```python
from build123d import *

# Parameters (mm, degrees)
SKETCH1_W           = 212.5
SKETCH1_H           = 339.725
SKETCH1_R           = 3.175
BOSS_EXTRUDE1_DEPTH = 3.175
CUT_EXTRUDE1_DEPTH  = 401.72360331
SKETCH3_R           = 4
CUT_EXTRUDE2_DEPTH  = 45.72
SKETCH4_R           = 4
CUT_EXTRUDE3_DEPTH  = 14.986


with BuildPart() as part:
    # Sketch1 → Boss-Extrude1 (new body)
    with BuildSketch(Plane(origin=(0, 0, 0), x_dir=(0, 0, -1), z_dir=(1, 0, 0))):
        with Locations((106.25, -169.8625)):
            Rectangle(SKETCH1_W, SKETCH1_H)
        with Locations((12.7, -12.7)):
            Circle(SKETCH1_R, mode=Mode.SUBTRACT)
        with Locations((199.8, -12.7)):
            Circle(SKETCH1_R, mode=Mode.SUBTRACT)
        with Locations((66.25, -35.2425)):
            Circle(SKETCH1_R, mode=Mode.SUBTRACT)
        with Locations((146.25, -35.2425)):
            Circle(SKETCH1_R, mode=Mode.SUBTRACT)
        with Locations((176.25, -57.8625)):
            Circle(SKETCH1_R, mode=Mode.SUBTRACT)
        with Locations((36.25, -57.8625)):
            Circle(SKETCH1_R, mode=Mode.SUBTRACT)
        with Locations((191.25, -104.5325)):
            Circle(SKETCH1_R, mode=Mode.SUBTRACT)
        with Locations((36.25, -169.8625)):
            Circle(SKETCH1_R, mode=Mode.SUBTRACT)
        with Locations((191.25, -169.8625)):
            Circle(SKETCH1_R, mode=Mode.SUBTRACT)
        with Locations((36.25, -281.8625)):
            Circle(SKETCH1_R, mode=Mode.SUBTRACT)
        with Locations((66.25, -304.4825)):
            Circle(SKETCH1_R, mode=Mode.SUBTRACT)
        with Locations((12.7, -327.025)):
            Circle(SKETCH1_R, mode=Mode.SUBTRACT)
        with Locations((199.8, -327.025)):
            Circle(SKETCH1_R, mode=Mode.SUBTRACT)
        with Locations((146.25, -304.4825)):
            Circle(SKETCH1_R, mode=Mode.SUBTRACT)
        with Locations(Location((191.25, -235.1925, 0), (0, 0, 180))):
            Circle(SKETCH1_R, mode=Mode.SUBTRACT)
    extrude(amount=BOSS_EXTRUDE1_DEPTH)

    # Sketch2 → Cut-Extrude1 (cut, through all)
    with BuildSketch(Plane(origin=(3.175, 0, 0), x_dir=(0, 0, -1), z_dir=(1, 0, 0))):
        with BuildLine():
            Line((165.85, -88.161695758), (165.85, -251.563304242))
            ThreePointArc((165.85, -251.563304242), (164.516472011, -257.22840036), (160.795934799, -261.703801323))
            Line((160.795934799, -261.703801323), (125.904065201, -288.012271))
            ThreePointArc((125.904065201, -288.012271), (122.183527989, -292.487671963), (120.85, -298.152768081))
            Line((120.85, -298.152768081), (120.85, -314.325))
            ThreePointArc((120.85, -314.325), (117.130256121, -323.305256121), (108.15, -327.025))
            Line((108.15, -327.025), (104.35, -327.025))
            ThreePointArc((104.35, -327.025), (95.369743879, -323.305256121), (91.65, -314.325))
            Line((91.65, -314.325), (91.65, -298.152768081))
            ThreePointArc((91.65, -298.152768081), (90.316472011, -292.487671963), (86.595934799, -288.012271))
            Line((86.595934799, -288.012271), (48.147303392, -259.022002919))
            ThreePointArc((48.147303392, -259.022002919), (44.532850149, -257.119362682), (40.501368593, -256.4625))
            Line((40.501368593, -256.4625), (25.4, -256.4625))
            ThreePointArc((25.4, -256.4625), (16.419743879, -252.742756121), (12.7, -243.7625))
            Line((12.7, -243.7625), (12.7, -207.9625))
            ThreePointArc((12.7, -207.9625), (16.419743879, -198.982243879), (25.4, -195.2625))
            Line((25.4, -195.2625), (48.95, -195.2625))
            ThreePointArc((48.95, -195.2625), (57.930256121, -191.542756121), (61.65, -182.5625))
            Line((61.65, -182.5625), (61.65, -157.1625))
            ThreePointArc((61.65, -157.1625), (57.930256121, -148.182243879), (48.95, -144.4625))
            Line((48.95, -144.4625), (25.4, -144.4625))
            ThreePointArc((25.4, -144.4625), (16.419743879, -140.742756121), (12.7, -131.7625))
            Line((12.7, -131.7625), (12.7, -95.9625))
            ThreePointArc((12.7, -95.9625), (16.419743879, -86.982243879), (25.4, -83.2625))
            Line((25.4, -83.2625), (40.501368593, -83.2625))
            ThreePointArc((40.501368593, -83.2625), (44.532850149, -82.605637318), (48.147303392, -80.702997081))
            Line((48.147303392, -80.702997081), (86.595934799, -51.712729))
            ThreePointArc((86.595934799, -51.712729), (90.316472011, -47.237328037), (91.65, -41.572231919))
            Line((91.65, -41.572231919), (91.65, -25.4))
            ThreePointArc((91.65, -25.4), (95.369743879, -16.419743879), (104.35, -12.7))
            Line((104.35, -12.7), (108.15, -12.7))
            ThreePointArc((108.15, -12.7), (117.130256121, -16.419743879), (120.85, -25.4))
            Line((120.85, -25.4), (120.85, -41.572231919))
            ThreePointArc((120.85, -41.572231919), (122.183527989, -47.237328037), (125.904065201, -51.712729))
            Line((125.904065201, -51.712729), (160.795934799, -78.021198677))
            ThreePointArc((160.795934799, -78.021198677), (164.516472011, -82.49659964), (165.85, -88.161695758))
        make_face()
    extrude(amount=-CUT_EXTRUDE1_DEPTH, mode=Mode.SUBTRACT)

    # Sketch3 → Cut-Extrude2 (cut)
    with BuildSketch(Plane.ZY):
        with Locations((-353.343139499, -302.41374809)):
            Circle(SKETCH3_R)
    extrude(amount=-CUT_EXTRUDE2_DEPTH, mode=Mode.SUBTRACT)

    # Sketch4 → Cut-Extrude3 (cut)
    with BuildSketch(Plane.ZY):
        with Locations((-76.9625, -23.613540107)):
            Circle(SKETCH4_R)
    extrude(amount=-CUT_EXTRUDE3_DEPTH, mode=Mode.SUBTRACT)


solid = part.part
```
Source: CAD feature listing. Evaluate the final solid. Frame: model axes, mm. A direction names the side the tool comes from. Coordinates: 2 decimals unless noted, no trailing zeros. Loops run counter-clockwise (first coordinate to the right, second up) from the corner with the lowest first, then second, coordinate; pieces in that order, holes last. Notation, with made-up numbers: (-35, 51.25) -> (-2, 51.25) arc R12 ccw to (-2, 55.25) -> close; hole circle Ø10 at (83.25, 5). An arc over 180 degrees is marked (long way). One line per item, written item: value. Start each with the question number.
Q1. Set-up query: faces 1 (the face through (1.61, -16.32, -117.03)), 2 (the face through (0, -167, -58)). Return all of +Z, -Z, +X, -X, +Y, -Y with unobstructed straight access to the full face (end or side cutting, diameter ignored); none if empty.
Q2. Section query B-B, the plane x = 1.3. Give the number of separate pieces and of enclosed holes in the cut face, and give its area (3 significant figures).
Q3. Mould query, pull axis Z, two halves, no side actions, for faces 3 (the face through (1.57, -104.39, -188.08)), 4 (the face through (3.175, -167, -58)). Classes: pulls with the +Z half, pulls with the -Z half, needs draft (parallel to the pull), parting line crosses it, or undercut.
Q4. Contact query for a flat-ended pin moving along its axis: P1, Ø4, axis at y = -281.86, z = -36.25, coming from the -X side. Output: stop coordinate, or through.
Q5. Section query A-A, the plane z = -130.5. Return the cut outline in (x, y) (3 decimals), and give its area (3 significant figures).
Q6. Line query: line 1 along Y through (x, z) = (1.6, -199.8) (3 decimals); line 2 along Z through (x, y) = (0.8, -175); line 3 along Y through (x, z) = (2.7, -40.5) (1 decimal). Output: solid intervals per line, ascending.
Results:
1. face 1: +X, -X
1. face 2: +Z, -Z, -X, +Y, -Y
2. separate pieces: 1
2. enclosed holes: 17
2. area: 40,400 mm^2
3. face 3: undercut
3. face 4: needs draft
4. P1: through
5. outline: (0, -339.725) -> (3.175, -339.725) -> (3.175, -284.547) -> (0, -284.547) -> close; (0, -55.178) -> (3.175, -55.178) -> (3.175, 0) -> (0, 0) -> close
5. area: 350 mm^2
6. line 1: -339.725 to -330.2, -323.85 to -15.875, -9.525 to 0
6. line 2: -212.5 to -165.85, -61.65 to 0
6. line 3: -339.7 to -256.5, -195.3 to -144.5, -83.3 to 0
